```python
from build123d import *

# Parameters (mm, degrees)
SKETCH1_W           = 420
SKETCH1_H           = 220
BOSS_EXTRUDE1_DEPTH = 10
SKETCH2_R           = 2.25
CUT_EXTRUDE1_DEPTH  = 10
SKETCH3_R           = 4
CUT_EXTRUDE2_DEPTH  = 4
CHAMFER1_SIZE       = 2
SKETCH5_W           = 4
SKETCH5_H           = 46
CUT_EXTRUDE3_DEPTH  = 116.38
SKETCH7_R           = 2.15
CUT_EXTRUDE4_DEPTH  = 11
SKETCH8_R           = 4
CUT_EXTRUDE5_DEPTH  = 4


with BuildPart() as part:
    # Sketch1 → Boss-Extrude1 (new body)
    with BuildSketch(Plane.XY):
        Rectangle(SKETCH1_W, SKETCH1_H)
    extrude(amount=BOSS_EXTRUDE1_DEPTH)

    # Sketch2 → Cut-Extrude1 (cut)
    with BuildSketch(Plane.XY.offset(10)):
        with Locations((-200, 60)):
            Circle(SKETCH2_R)
        with Locations((200, 60)):
            Circle(SKETCH2_R)
        with Locations((200, -100)):
            Circle(SKETCH2_R)
        with Locations((-200, -100)):
            Circle(SKETCH2_R)
    extrude(amount=-CUT_EXTRUDE1_DEPTH, mode=Mode.SUBTRACT)

    # Sketch3 → Cut-Extrude2 (cut)
    with BuildSketch(Plane.XY.offset(10)):
        with Locations((-200, 60)):
            Circle(SKETCH3_R)
        with Locations((-200, -100)):
            Circle(SKETCH3_R)
        with Locations((200, 60)):
            Circle(SKETCH3_R)
        with Locations((200, -100)):
            Circle(SKETCH3_R)
    extrude(amount=-CUT_EXTRUDE2_DEPTH, mode=Mode.SUBTRACT)

    # Chamfer1
    chamfer1_edges = [part.edges().sort_by_distance(p)[0] for p in [
        (210, -110, 5),
        (-210, -110, 5),
        (-210, 110, 5),
        (210, 110, 5),
    ]]
    chamfer(chamfer1_edges, length=CHAMFER1_SIZE)

    # Sketch5 → Cut-Extrude3 (cut)
    with BuildSketch(Plane(origin=(210, 0, 0), x_dir=(0, 0, -1), z_dir=(1, 0, 0))):
        with Locations((-8, 66)):
            Rectangle(SKETCH5_W, SKETCH5_H)
    extrude(amount=-CUT_EXTRUDE3_DEPTH, mode=Mode.SUBTRACT)

    # Sketch7 → Cut-Extrude4 (cut, through all)
    with BuildSketch(Plane.XY.offset(10)):
        with Locations((200, -90)):
            Circle(SKETCH7_R)
        with Locations((200, 70)):
            Circle(SKETCH7_R)
        with Locations((-200, -90)):
            Circle(SKETCH7_R)
        with Locations((-200, 70)):
            Circle(SKETCH7_R)
    extrude(amount=-CUT_EXTRUDE4_DEPTH, mode=Mode.SUBTRACT)

    # Sketch8 → Cut-Extrude5 (cut)
    with BuildSketch(Plane.XY.offset(10)):
        with Locations((-200, 70)):
            Circle(SKETCH8_R)
        with Locations((-200, -90)):
            Circle(SKETCH8_R)
        with Locations((200, -90)):
            Circle(SKETCH8_R)
    extrude(amount=-CUT_EXTRUDE5_DEPTH, mode=Mode.SUBTRACT)


solid = part.part
```
Read the model definition and answer for the solid it produces. Units are mm, in the model's axes. A direction names the side the tool comes from. Coordinates: 2 decimals unless noted, no trailing zeros. Return JSON: item names as keys, results as strings.
1. Determine the mould class of faces 4 (the face through (-198.154, 56.451, 8.028)), 5 (the face through (-210, -2, 5)), 6 (the face through (-3, 110, 5)) for opening direction Y: pulls with the +Y half, pulls with the -Y half, needs draft (parallel to the pull), parting line crosses it, or undercut.
Found:
{"face 4": "undercut", "face 5": "needs draft", "face 6": "pulls with the +Y half"}
2. Find the intervals of material crossed by line 1 along Y through (x, z) = (-200, 9.2); line 2 along Y through (x, z) = (200, 3); line 3 along Y through (x, z) = (200, 9.05), in increasing order. Write a range as from..to.
Found:
{"line 1": "-110..-104, -96..-94, -86..56, 64..66, 74..110", "line 2": "-110..-102.25, -97.75..-92.15, -87.85..57.75, 62.25..67.85, 72.15..110", "line 3": "-110..-104, -96..-94, -86..43, 89..110"}
3. This flat-tipped pin is pushed along its axis until it touches: P1, Ø23, axis at x = 139, y = 60.5, coming from the +Z side. Where does it stop, or does it pass through?
Found:
{"P1": "z = 6"}
4. A tool of negligible diameter and unlimited length cuts with its end or side. For faces 1 (the face through (153, 66, 6)), 2 (the face through (-3, 2, 0)), 3 (the face through (202, -92, 6)), from which of +Z, -Z, +X, -X, +Y, -Y can it reach the whole face along a straight path? Write none if from no direction.
Found:
{"face 1": "+Z, +X", "face 2": "-Z, +X, -X, +Y, -Y", "face 3": "+Z"}
